Read the model definition and answer for the solid it produces. Units are mm, in the model's axes. Face numbers are marked on the shaded views. A direction names the side the tool comes from. Round coordinates to 2 decimals unless told otherwise and drop trailing zeros. Write each loop counter-clockwise with the first axis right and the second up, starting at its lowest first coordinate (ties: lowest second). Pieces come first, ordered by that corner, then holes. Notation, with made-up numbers: (13.5, -34.75) -> (19.5, -34.75) arc R10 ccw to (19.5, -27.75) -> close; hole circle Ø3 at (-8, -6). An arc over 180 degrees is marked (long way). Return JSON: item names as keys, results as strings.
Autodesk Inventor part; units mm, degrees
ref_plane "YZ Plane" through (0, 0, 0) normal (1, 0, 0) x (0, 1, 0)
ref_plane "XZ Plane" through (0, 0, 0) normal (0, 1, 0) x (-1, 0, 0)
ref_plane "XY Plane" through (0, 0, 0) normal (0, 0, 1) x (1, 0, 0)
sketch "Sketch1" plane through (0, 0, 0) normal (0, 1, 0) x (-1, 0, 0)
  line L0 (0, 0) -> (95, 0)
  line L1 (95, 0) -> (95, -65)
  line L2 (95, -65) -> (0, -65)
  line L3 (0, -65) -> (0, 0)
  line L4 (98, -68) -> (98, 3)
  line L5 (98, 3) -> (-3, 3)
  line L6 (-3, 3) -> (-3, -68)
  line L7 (-3, -68) -> (98, -68)
  dimension "d0" = 95
  dimension "d1" = 65
  dimension "d2" = 3
extrude "Extrusion1" add sketch "Sketch1" along normal blind 32 contours L0 L1 L2 L3 | L7 L6 L5 L4
sketch "Sketch2" plane through (0, 32, 0) normal (0, 1, 0) x (1, 0, 0)
  line L0 (0, 0) -> (-95, 0)
  line L1 (-95, 0) -> (-95, 65)
  line L2 (-95, 65) -> (0, 65)
  line L3 (0, 65) -> (0, 0)
  dimension "d5" = 95
  dimension "d6" = 65
extrude "Extrusion2" cut sketch "Sketch2" against normal blind 30
sketch "Sketch3" plane through (0, 2, 0) normal (0, 1, 0) x (1, 0, 0)
  line L0 (0, 65) -> (0, 0)
  line L1 (0, 0) -> (0, 9)
  line L2 (0, 9) -> (-10, 9)
  circle A0 centre (-10, 9) radius 2
  circle A1 centre (-10, 9) radius 4
  circle A2 centre (-10, 58) radius 4
  circle A3 centre (-10, 58) radius 2
  circle A4 centre (-68, 9) radius 4
  circle A5 centre (-68, 9) radius 2
  circle A6 centre (-68, 58) radius 4
  circle A7 centre (-68, 58) radius 2
  dimension "d9" = 9
  dimension "d10" = 10
  dimension "d11" = 4
  dimension "d12" = 8
  dimension "d15" = 49
  dimension "d18" = 58
extrude "Extrusion3" add sketch "Sketch3" along normal blind 5
sketch "Sketch4" plane through (0, 32, 0) normal (0, 1, 0) x (1, 0, 0)
  line L0 (3, 68) -> (-98, 68)
  line L1 (3, 68) -> (-98, 68)
  line L2 (-98, 68) -> (-98, 81)
  line L3 (-98, 81) -> (3, 81)
  line L4 (3, 81) -> (3, 68)
  point P0 (0, 0)
  dimension "d23" = 13
  dimension "d62" = 101
extrude "Extrusion4" add sketch "Sketch4" against normal blind 3
sketch "Sketch5" plane through (0, 32, 0) normal (0, 1, 0) x (1, 0, 0)
  line L0 (-98, 81) -> (3, 81)
  line L1 (3, 81) -> (-97, 81)
  line L2 (-97, 81) -> (-97, 78)
  line L3 (-97, 78) -> (3, 78)
  line L4 (3, 78) -> (3, 81)
  line L5 (3, 81) -> (0, 81)
  line L6 (0, 81) -> (0, -3)
  line L7 (0, -3) -> (3, -3)
  line L8 (3, -3) -> (3, 81)
  line L9 (-98, 68) -> (-98, 81)
  line L10 (-98, 81) -> (-95, 81)
  line L11 (-95, 81) -> (-95, -3)
  line L12 (-95, -3) -> (-98, -3)
  line L13 (-98, -3) -> (-98, 81)
  line L14 (-98, -3) -> (2, -3)
  line L15 (2, -3) -> (2, 0)
  line L16 (2, 0) -> (-98, 0)
  line L17 (-98, 0) -> (-98, -3)
  point P0 (0, 0)
  dimension "d26" = 100
  dimension "d27" = 3
  dimension "d28" = 3
  dimension "d29" = 84
  dimension "d30" = 3
  dimension "d31" = 84
  dimension "d32" = 100
  dimension "d33" = 3
extrude "Extrusion5" add sketch "Sketch5" along normal blind 26 contours L0 L2 L3 L11 L16 L13 L9 | L0 L11 L3 L2 | L0 L6 L3 L11 | L16 L11 L12 L13 | L0 L4 L3 L6 | L16 L6 L14 L11 | L3 L8 L7 L15 L16 L6 | L16 L15 L7 L6
sketch "Sketch6" plane through (-98, 0, -68) normal (-1, 0, 0) x (0, 0, 1)
  line L0 (71, 0) -> (71, 32)
  line L1 (71, 58) -> (61.858, 58)
  line L2 (71, 58) -> (-13, 58)
  line L3 (61.858, 58) -> (61.858, 51.5)
  line L4 (61.858, 51.5) -> (11.858, 51.5)
  line L5 (11.858, 51.5) -> (11.858, 36.5)
  line L6 (11.858, 36.5) -> (61.858, 36.5)
  line L7 (61.858, 36.5) -> (61.858, 51.5)
  line L8 (3, 32) -> (3, 2)
  line L9 (3, 2) -> (3, 7)
  line L10 (68, 2) -> (3, 2)
  line L11 (3, 2) -> (8, 2) construction
  line L12 (3, 7) -> (8.54, 7)
  line L13 (8.54, 7) -> (22.54, 7)
  line L14 (22.54, 7) -> (22.54, 25)
  line L15 (22.54, 25) -> (8.54, 25)
  line L16 (8.54, 25) -> (8.54, 7)
  line L17 (22.54, 7) -> (27.04, 7)
  line L18 (27.04, 7) -> (41.04, 7)
  line L19 (41.04, 7) -> (41.04, 25)
  line L20 (41.04, 25) -> (27.04, 25)
  line L21 (27.04, 25) -> (27.04, 7)
  point P0 (68, 0)
  dimension "d36" = 9.142
  dimension "d37" = 6.5
  dimension "d38" = 50
  dimension "d39" = 15
  dimension "d40" = 5
  dimension "d41" = 90
  dimension "d42" = 5.54
  dimension "d43" = 14
  dimension "d44" = 18
  dimension "d45" = 4.5
  dimension "d46" = 14
  dimension "d47" = 18
extrude "Extrusion6" cut sketch "Sketch6" against normal blind 3
sketch "Sketch7" plane through (3, 0, -68) normal (0, 0, -1) x (-1, 0, 0)
  line L0 (3, 2) -> (3, 32)
  line L1 (3, 2) -> (4, 2)
  line L2 (4, 2) -> (4, 7)
  line L3 (4, 7) -> (31.75, 7)
  line L4 (31.75, 7) -> (39.75, 7)
  line L5 (39.75, 7) -> (39.75, 11)
  line L6 (39.75, 11) -> (31.75, 11)
  line L7 (31.75, 11) -> (31.75, 7)
  point P0 (3, 0)
  point P1 (3, 58)
  dimension "d50" = 1
  dimension "d51" = 5
  dimension "d52" = 27.75
  dimension "d53" = 8
  dimension "d54" = 4
extrude "Extrusion7" cut sketch "Sketch7" against normal blind 3
sketch "Sketch8" plane through (-98, 0, 3) normal (0, 0, 1) x (1, 0, 0)
  line L0 (101, 0) -> (101, 29)
  line L1 (101, 0) -> (101, 20)
  line L2 (101, 20) -> (86, 20)
  line L3 (86, 20) -> (16, 20)
  circle A0 centre (86, 20) radius 1.75
  circle A1 centre (16, 20) radius 1.75
  point P0 (98, 0)
  dimension "d63" = 20
  dimension "d64" = 15
  dimension "d65" = 70
  dimension "d66" = 3.5
  dimension "d67" = 3.5
extrude "Extrusion8" cut sketch "Sketch8" against normal blind 10
properties part number "MainPCB_RPI_Case"
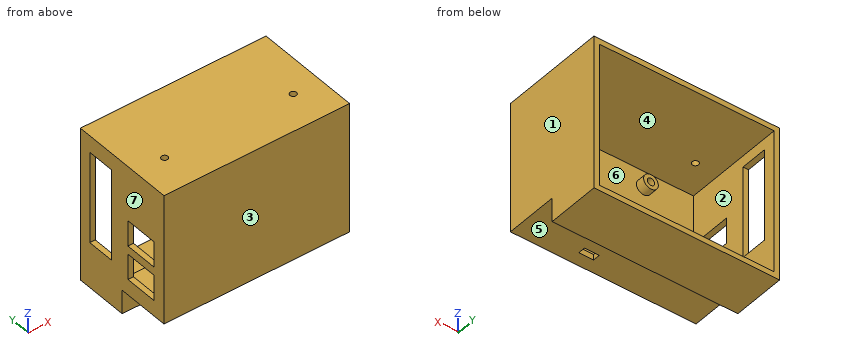
Item 1: For a pull along X with two mould halves and no side action, classify the marked faces 1, 2, 3 and 4 as released by +X, released by -X, zero draft, split by the parting line, or undercut.
Worked answers:
{"face 1": "released by +X", "face 2": "undercut", "face 3": "zero draft", "face 4": "undercut"}
Item 2: Section C-C (z = -58) is taken. Give the vertices of the cut face in (x, y).
Worked answers:
{"outline": "(-98, 0) -> (3, 0) -> (3, 58) -> (0, 58) -> (0, 2) -> (-6, 2) -> (-6, 7) -> (-8, 7) -> (-8, 2) -> (-12, 2) -> (-12, 7) -> (-14, 7) -> (-14, 2) -> (-64, 2) -> (-64, 7) -> (-66, 7) -> (-66, 2) -> (-70, 2) -> (-70, 7) -> (-72, 7) -> (-72, 2) -> (-95, 2) -> (-95, 7) -> (-98, 7) -> close; (-98, 25) -> (-95, 25) -> (-95, 58) -> (-98, 58) -> close"}
Item 3: Straight lines are drawn through the part: L1, parallel to X at y = 5.3, z = -58; L2, parallel to Z at x = -10, y = 4.8; L3, parallel to X at y = 30, z = -3. For each, find the intervals that lie inside material, in ascending order. Write a range as [from, to].
Worked answers:
{"L1": "x = [-98, -95], [-72, -70], [-66, -64], [-14, -12], [-8, -6], [0, 3]", "L2": "z = [-68, -65], [-62, -60], [-56, -54], [-13, -11], [-7, -5], [0, 3]", "L3": "x = [-98, -95], [0, 3]"}
Item 4: Flat-ended cylindrical pins translate along their axes: pin 1 (14.5 mm diameter, centred on x = -54.5, z = -76, fed in from -Y); pin 2 (2.5 mm diameter, centred on x = -67.5, z = -60, fed in from +Y); pin 3 (1.2 mm diameter, centred on x = -67.5, z = -9, fed in from +Y). Find the tip coordinate at first contact, or state that the pin passes through.
Worked answers:
{"pin 1": "stops at y = 29", "pin 2": "stops at y = 7", "pin 3": "stops at y = 2"}
Item 5: Section D-D (x = -24) is taken. Give the vertices of the cut face in (y, z).
Worked answers:
{"outline": "(0, -68) -> (29, -68) -> (29, -81) -> (58, -81) -> (58, -78) -> (32, -78) -> (32, -65) -> (2, -65) -> (2, 0) -> (58, 0) -> (58, 3) -> (0, 3) -> close"}
Item 6: Section A-A (y = 13) is taken. Give the vertices of the cut face in (x, z), then the cut area to 3 significant figures.
Worked answers:
{"outline": "(-98, -68) -> (3, -68) -> (3, 3) -> (-98, 3) -> (-98, -26.96) -> (-95, -26.96) -> (-95, 0) -> (0, 0) -> (0, -65) -> (-95, -65) -> (-95, -59.46) -> (-98, -59.46) -> close; (-98, -45.46) -> (-95, -45.46) -> (-95, -40.96) -> (-98, -40.96) -> close", "area": "912 mm2"}
Item 7: A tool of negligible diameter and unlimited length cuts with its end or side. For the marked faces 5, 6 and 7, from which of +Z, -Z, +X, -X, +Y, -Y can it reach the whole face along a straight path? Write none if from no direction.
Worked answers:
{"face 5": "-Z, +X, -X, -Y", "face 6": "+Y", "face 7": "+Z, -Z, -X, +Y, -Y"}
Item 8: Section B-B (y = 20) is taken. Give the vertices of the cut face in (x, z), then the cut area to 3 significant figures.
Worked answers:
{"outline": "(-98, -68) -> (3, -68) -> (3, 3) -> (-10.25, 3) -> (-10.25, 0) -> (0, 0) -> (0, -65) -> (-95, -65) -> (-95, -59.46) -> (-98, -59.46) -> close; (-98, -45.46) -> (-95, -45.46) -> (-95, -40.96) -> (-98, -40.96) -> close; (-98, -26.96) -> (-95, -26.96) -> (-95, 0) -> (-83.75, 0) -> (-83.75, 3) -> (-98, 3) -> close; (-80.25, 0) -> (-13.75, 0) -> (-13.75, 3) -> (-80.25, 3) -> close", "area": "891 mm2"}
